Could you check a few things on this model? Use its own coordinates, in mm. A direction names the side the tool comes from. Coordinates: 2 decimals unless noted, no trailing zeros. Loops run counter-clockwise (first coordinate to the right, second up) from the corner with the lowest first, then second, coordinate; pieces in that order, holes last. Notation, with made-up numbers: (82, -15) - (135, -15) arc R23 ccw to (135, 0) - close; hole circle Ø10 at (27.5, 19). An arc over 180 degrees is marked (long way). One line per item, written item: value. Start each with the question number.
(1) If we section it at B-B on x = 23.5: Write out the boundary of the cut face in (y, z).
(2) If we mould it in two halves opening along X, with no side actions, what happens to faces 1 (the face through (50, 2, -4)), 2 (the face through (2.46, 9.76, 2.17)), 3 (the face through (68.393, 0.554, 0.723))? For each: pulls with the +X half, pulls with the -X half, needs draft (parallel to the pull), parting line crosses it, or undercut.
(3) If we section it at A-A on x = 46: Write out the boundary of the cut face in (y, z), then the cut area to 3 significant figures.
(4) If I drill on line 1 along X through (y, z) = (-5.5, -4); line 2 along Y through (x, z) = (2.5, 0); line 3 along X through (y, z) = (4.5, -4.75), over which ranges is the centre line in solid material (lowest first)? Write a range as from..to.
(5) I'm going to push flat-ended pins straight in: P1, Ø1, axis at x = 13, y = -1.5, coming from the -Z side; P2, Ø2, axis at x = 58.5, y = 1.5, coming from the -Z side; P3, Ø3, axis at y = -1.5, z = -1.5, coming from the +X side; P4, Ø1.5, axis at y = -4.5, z = 1, coming from the -X side. Where does each tip first touch, or does it pass through?
(6) On a 3-axis mill with a long thin cutter (end or side, diameter ignored), from which of +Z, -Z, +X, -X, +Y, -Y can I reach the whole of each face in a straight line? I mean faces 4 (the face through (48.48, 7.81, 1.73)), 5 (the face through (63.63, 0.591, -1.426)), 6 (the face through (0, 0, 0)). Say none if no direction works.
```python
from build123d import *


with BuildPart() as part:
    # Sketch 153 → Повернуть1 (revolve)
    with BuildSketch(Plane(origin=(0, 0, 0), x_dir=(1, 0, 0), z_dir=(0, 1, 0))):
        Polygon((0, 10), (0, 0), (1, 0), (1, 5.25), (3.5, 5.25), (3.5, 0), (5, 0), (5, 10), align=None)
        with BuildLine():
            ThreePointArc((7, 8), (6.414213562, 9.414213562), (5, 10))
            Line((5, 10), (5, 0))
            Line((5, 0), (7, 0))
            Line((7, 0), (7, 8))
        make_face()
        with BuildLine():
            ThreePointArc((10.2, 4.8), (9.2627417, 7.0627417), (7, 8))
            Line((7, 8), (7, 0))
            Line((7, 0), (10.2, 0))
            Line((10.2, 0), (10.2, 4.8))
        make_face()
    revolve(axis=Axis((5, 0, 0), (-1, 0, 0)))

    # Sketch 880 → Повернуть2 (revolve)
    with BuildSketch(Plane(origin=(0, 0, 0), x_dir=(1, 0, 0), z_dir=(0, 1, 0))):
        with BuildLine():
            Line((10.2, 4.8), (10.2, 0))
            Line((10.2, 0), (70.4, 0))
            Line((70.4, 0), (65.331156927, 2.3))
            Line((65.331156927, 2.3), (63.30687842, 1.4))
            Line((63.30687842, 1.4), (62.3, 1.4))
            Line((62.3, 1.4), (62.3, 5.291657255))
            ThreePointArc((62.3, 5.291657255), (60.748015293, 6.979485771), (58.457233587, 7.07818129))
            Line((58.457233587, 7.07818129), (50, 4))
            Line((50, 4), (50, 8))
            Line((50, 8), (47, 8))
            ThreePointArc((47, 8), (44.7372583, 7.0627417), (43.8, 4.8))
            ThreePointArc((43.8, 4.8), (27, 2.591400685), (10.2, 4.8))
        make_face()
    revolve(axis=Axis((50, 0, 0), (-1, 0, 0)))


solid = part.part
```
Values:
1. outline: circle Ø5.37 at (0, 0)
2. face 1: undercut
2. face 2: needs draft
2. face 3: pulls with the +X half
3. outline: circle Ø15.68 at (0, 0)
3. area: 193 mm2
4. line 1: x = 0..9.5, 44.5..50, 57.69..61.08
4. line 2: y = -10..-5.25, 5.25..10
4. line 3: x = 0..9.68, 44.32..50, 56.99..61.43
5. P1: stops at z = -4.04
5. P2: stops at z = -7.2
5. P3: stops at x = 69.03
5. P4: stops at x = 0
6. face 4: +X
6. face 5: none
6. face 6: +Z, -Z, -X, +Y, -Y
